from build123d import *

# Parameters (mm, degrees)
SKETCH1_R           = 4.75
BOSS_EXTRUDE1_DEPTH = 0.85
SKETCH3_R           = 3.5
BOSS_EXTRUDE3_DEPTH = 3.15
SKETCH4_R           = 1
CUT_EXTRUDE1_DEPTH  = 4
SKETCH5_R           = 2.75
SKETCH5_R_2         = 1.75
CUT_EXTRUDE2_DEPTH  = 0.2
SKETCH6_R           = 2.75
SKETCH6_R_2         = 1.75
CUT_EXTRUDE3_DEPTH  = 0.2


with BuildPart() as part:
    # Sketch1 → Boss-Extrude1 (new body)
    with BuildSketch(Plane.XY):
        Circle(SKETCH1_R)
    extrude(amount=BOSS_EXTRUDE1_DEPTH)

    # Sketch3 → Boss-Extrude3 (add)
    with BuildSketch(Plane.XY.offset(0.85)):
        Circle(SKETCH3_R)
    extrude(amount=BOSS_EXTRUDE3_DEPTH)

    # Sketch4 → Cut-Extrude1 (cut)
    with BuildSketch(Plane.XY.offset(4)):
        Circle(SKETCH4_R)
    extrude(amount=-CUT_EXTRUDE1_DEPTH, mode=Mode.SUBTRACT)

    # Sketch5 → Cut-Extrude2 (cut)
    with BuildSketch(Plane.XY.offset(4)):
        Circle(SKETCH5_R)
        Circle(SKETCH5_R_2, mode=Mode.SUBTRACT)
    extrude(amount=-CUT_EXTRUDE2_DEPTH, mode=Mode.SUBTRACT)

    # Sketch6 → Cut-Extrude3 (cut)
    with BuildSketch(Plane(origin=(0, 0, 0), x_dir=(-1, 0, 0), z_dir=(0, 0, -1))):
        Circle(SKETCH6_R)
        Circle(SKETCH6_R_2, mode=Mode.SUBTRACT)
    extrude(amount=-CUT_EXTRUDE3_DEPTH, mode=Mode.SUBTRACT)


solid = part.part
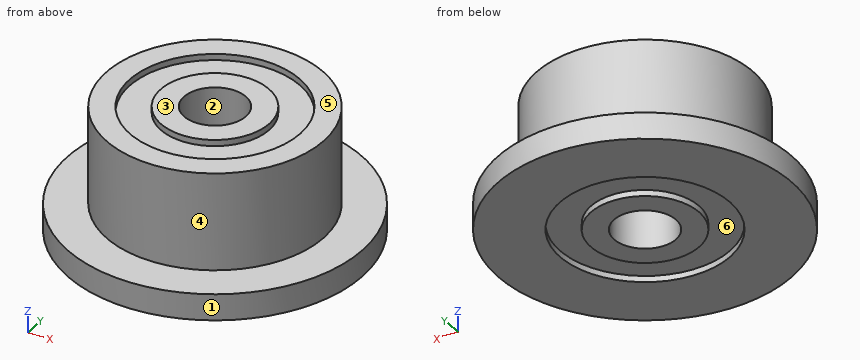
Build history of the part. All positions in model axes, mm. Face numbers are marked on the shaded views. A direction names the side the tool comes from. Coordinates: 2 decimals unless noted, no trailing zeros. Order: outer loops, then holes, each group sorted by start corner. A loop starts at its lowest first (then second) coordinate and runs counter-clockwise, first axis right, second up. Notation, with made-up numbers: (54, 55) -> (75, 55) arc R14 cw to (75, 70) -> close; hole circle Ø6 at (78.25, 49). An arc over 180 degrees is marked (long way). One line per item, written item: value.
(1) Mould opens along X. For the marked faces 1, 2 and 3 say: pulls with the +X half, pulls with the -X half, needs draft (parallel to the pull), parting line crosses it, or undercut.
Checked values:
face 1: parting line crosses it
face 2: undercut
face 3: needs draft
(2) Tool access for the marked faces 4, 5 and 6: list every direction of +Z, -Z, +X, -X, +Y, -Y with a clear straight run to the whole face (end or side of a thin tool).
Checked values:
face 4: +Z
face 5: +Z, +X, -X, +Y, -Y
face 6: -Z
(3) Slice it at A-A, the plane x = 0. List the corners of the cut face in (y, z), plus the area to 3 significant figures.
Checked values:
outline: (-4.75, 0) -> (-2.75, 0) -> (-2.75, 0.2) -> (-1.75, 0.2) -> (-1.75, 0) -> (-1, 0) -> (-1, 4) -> (-1.75, 4) -> (-1.75, 3.8) -> (-2.75, 3.8) -> (-2.75, 4) -> (-3.5, 4) -> (-3.5, 0.85) -> (-4.75, 0.85) -> close; (1, 0) -> (1.75, 0) -> (1.75, 0.2) -> (2.75, 0.2) -> (2.75, 0) -> (4.75, 0) -> (4.75, 0.85) -> (3.5, 0.85) -> (3.5, 4) -> (2.75, 4) -> (2.75, 3.8) -> (1.75, 3.8) -> (1.75, 4) -> (1, 4) -> close
area: 21.3 mm2
(4) Slice it at D-D, the plane x = -2.5. List the corners of the cut face in (y, z).
Checked values:
outline: (-4.04, 0) -> (-1.15, 0) -> (-1.15, 0.2) -> (1.15, 0.2) -> (1.15, 0) -> (4.04, 0) -> (4.04, 0.85) -> (2.45, 0.85) -> (2.45, 4) -> (1.15, 4) -> (1.15, 3.8) -> (-1.15, 3.8) -> (-1.15, 4) -> (-2.45, 4) -> (-2.45, 0.85) -> (-4.04, 0.85) -> close
(5) Slice it at C-C, the plane z = 1.4. List the corners of the cut face in (x, y).
Checked values:
outline: circle Ø7 at (0, 0); hole circle Ø2 at (0, 0)
(6) Probe line 1 (Y direction, x = 0, z = 0.15); line 2 (Y direction, x = 0, z = 2.6); line 3 (Z direction, x = 3.5, y = -2.25). List the from-to ranges inside material, lowest first. Write a range as [from, to].
Checked values:
line 1: [-4.75, -2.75], [-1.75, -1], [1, 1.75], [2.75, 4.75]
line 2: [-3.5, -1], [1, 3.5]
line 3: [0, 0.85]
